Geometry check sheet. Reference: drawing and pictorial views, mm from the part's lowest x, y, z. Round coordinates to 2 decimals unless told otherwise and drop trailing zeros. Order: outer loops, then holes, each group sorted by start corner. A loop starts at its lowest first (then second) coordinate and runs counter-clockwise, first axis right, second up.
Q1. Cross-section at C-C on y = 57.15. Record the cut outline in (x, z).
Q2. Cross-section at A-A on x = 19.05. Record the cut outline in (y, z), then the cut area to 3 significant figures.
Q3. Scan lines: probe 1 along Y at (x, z) = (57.15, 3.5); probe 2 along X at (y, z) = (59, 1.5); probe 3 along X at (y, z) = (19.5, 2.5). Record each from-to range of solid material in increasing order.
Q4. Cross-section at B-B on z = 3. Give the number of separate pieces and of enclosed holes in the cut face, then the cut area to 3 significant figures.
Q5. Depth check by flat-ended pin: P1, Ø2, axis at x = 41, z = 3.5, coming from the -Y side. Enter the tip coordinate at first touch or a pass-through.
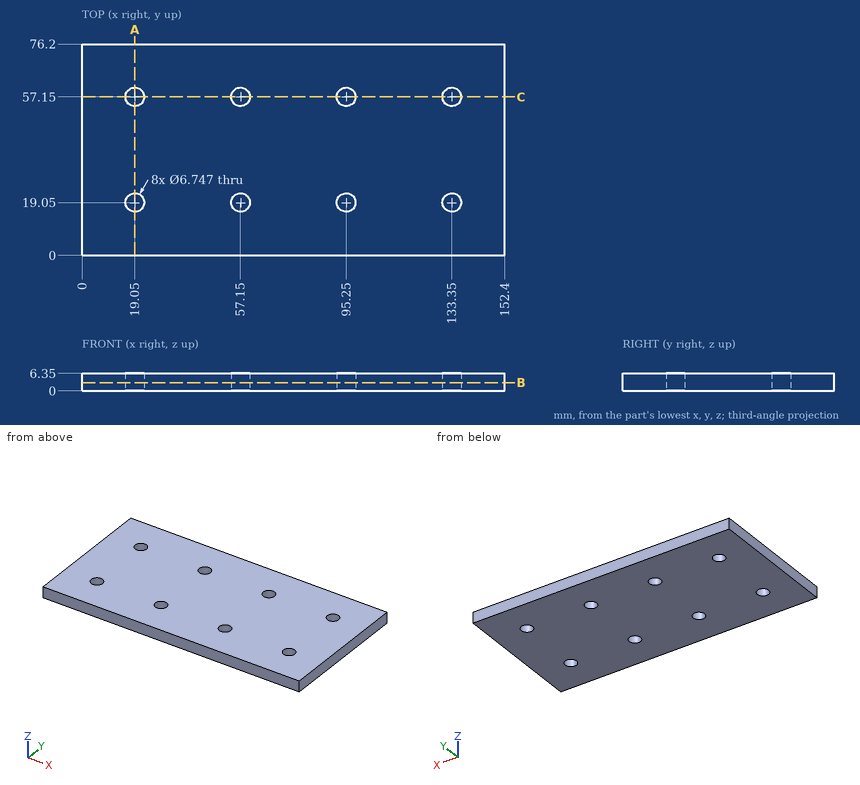
Results found:
1. outline: (0, 0) - (15.68, 0) - (15.68, 6.35) - (0, 6.35) - close; (22.42, 0) - (53.78, 0) - (53.78, 6.35) - (22.42, 6.35) - close; (60.52, 0) - (91.88, 0) - (91.88, 6.35) - (60.52, 6.35) - close; (98.62, 0) - (129.98, 0) - (129.98, 6.35) - (98.62, 6.35) - close; (136.72, 0) - (152.4, 0) - (152.4, 6.35) - (136.72, 6.35) - close
2. outline: (0, 0) - (15.68, 0) - (15.68, 6.35) - (0, 6.35) - close; (22.42, 0) - (53.78, 0) - (53.78, 6.35) - (22.42, 6.35) - close; (60.52, 0) - (76.2, 0) - (76.2, 6.35) - (60.52, 6.35) - close
2. area: 398 mm2
3. probe 1: y = 0 to 15.68, 22.42 to 53.78, 60.52 to 76.2
3. probe 2: x = 0 to 16.23, 21.87 to 54.33, 59.97 to 92.43, 98.07 to 130.53, 136.17 to 152.4
3. probe 3: x = 0 to 15.71, 22.39 to 53.81, 60.49 to 91.91, 98.59 to 130.01, 136.69 to 152.4
4. separate pieces: 1
4. enclosed holes: 8
4. area: 11,300 mm2
5. P1: stops at y = 0
